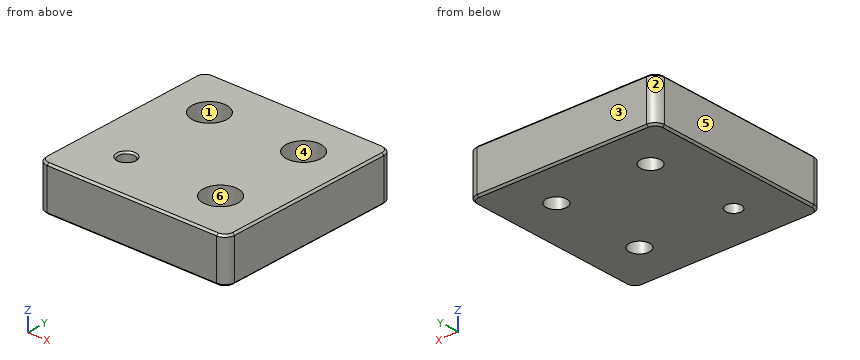
```python
from build123d import *

# Parameters (mm, degrees)
SKETCH1_W                                           = 60
SKETCH1_H                                           = 60
BOSS_EXTRUDE1_DEPTH                                 = 14
CBORE_FOR_M6_HEX_SOCKET_HEAD_CAP_SCREW1_D           = 6.5
CBORE_FOR_M6_HEX_SOCKET_HEAD_CAP_SCREW1_CBORE_D     = 11
CBORE_FOR_M6_HEX_SOCKET_HEAD_CAP_SCREW1_CBORE_DEPTH = 8
M6_TAPPED_HOLE1_D                                   = 5
M6_TAPPED_HOLE1_CSINK_D                             = 6.05
M6_TAPPED_HOLE1_CSINK_ANGLE                         = 90
FILLET1_R                                           = 3
CHAMFER1_SIZE                                       = 0.6


with BuildPart() as part:
    # Sketch1 → Boss-Extrude1 (new body)
    with BuildSketch(Plane.XY):
        Rectangle(SKETCH1_W, SKETCH1_H)
    extrude(amount=BOSS_EXTRUDE1_DEPTH)

    # CBORE for M6 Hex Socket Head Cap Screw1 (through all)
    with Locations(Plane.XY.offset(14)):
        with Locations((-15, 15), (15, 15), (15, -15)):
            CounterBoreHole(CBORE_FOR_M6_HEX_SOCKET_HEAD_CAP_SCREW1_D / 2, CBORE_FOR_M6_HEX_SOCKET_HEAD_CAP_SCREW1_CBORE_D / 2, CBORE_FOR_M6_HEX_SOCKET_HEAD_CAP_SCREW1_CBORE_DEPTH)

    # M6 Tapped Hole1 (through all)
    with Locations(Plane.XY.offset(14)):
        with Locations((-15, -15)):
            CounterSinkHole(M6_TAPPED_HOLE1_D / 2, M6_TAPPED_HOLE1_CSINK_D / 2, counter_sink_angle=M6_TAPPED_HOLE1_CSINK_ANGLE)

    # Fillet1
    fillet1_edges = [part.edges().sort_by_distance(p)[0] for p in [
        (-30, 30, 7),
        (30, 30, 7),
        (30, -30, 7),
        (-30, -30, 7),
    ]]
    fillet(fillet1_edges, radius=FILLET1_R)

    # Chamfer1
    chamfer1_edges = [part.edges().sort_by_distance(p)[0] for p in [
        (-30, 0, 0),
        (-30, 0, 14),
        (0, 30, 0),
        (30, 0, 0),
        (0, -30, 0),
        (-29.121320344, -29.121320344, 0),
        (29.121320344, -29.121320344, 0),
        (29.121320344, 29.121320344, 0),
        (-29.121320344, 29.121320344, 0),
        (0, 30, 14),
        (0, -30, 14),
        (30, 0, 14),
        (-29.121320344, -29.121320344, 14),
        (29.121320344, -29.121320344, 14),
        (29.121320344, 29.121320344, 14),
        (-29.121320344, 29.121320344, 14),
    ]]
    chamfer(chamfer1_edges, length=CHAMFER1_SIZE)


solid = part.part
```
Work out the finished part from the listing and answer in its coordinate system (mm). Face numbers are marked on the shaded views. A direction names the side the tool comes from. Round coordinates to 2 decimals unless told otherwise and drop trailing zeros. Loops run counter-clockwise (first coordinate to the right, second up) from the corner with the lowest first, then second, coordinate; pieces in that order, holes last.
(1) The mould has two halves that part along X. Classify the marked faces 3, 4, 5 and 6: pulls with the +X half, pulls with the -X half, needs draft (parallel to the pull), parting line crosses it, or undercut.
Computed values:
face 3: needs draft
face 4: undercut
face 5: pulls with the -X half
face 6: undercut
(2) Each of these flat-tipped pins is pushed along its axis until it touches: P1, Ø12, axis at x = 16, y = -13, coming from the +Z side; P2, Ø3.5, axis at x = -13, y = 15.5, coming from the +Z side. Where does it stop, or does it pass through?
Computed values:
P1: stops at z = 14
P2: stops at z = 6
(3) The part is cut by section A-A, the plane y = 15. Give the vertices of the cut face in (x, z), and give its area (3 significant figures).
Computed values:
outline: (-30, 0.6) - (-29.4, 0) - (-18.25, 0) - (-18.25, 6) - (-20.5, 6) - (-20.5, 14) - (-29.4, 14) - (-30, 13.4) - close; (-11.75, 0) - (11.75, 0) - (11.75, 6) - (9.5, 6) - (9.5, 14) - (-9.5, 14) - (-9.5, 6) - (-11.75, 6) - close; (18.25, 0) - (29.4, 0) - (30, 0.6) - (30, 13.4) - (29.4, 14) - (20.5, 14) - (20.5, 6) - (18.25, 6) - close
area: 585 mm2
(4) Find the intervals of material crossed by L1, parallel to Y at x = 15, z = 12; L2, parallel to Y at x = 15, z = 3.05; L3, parallel to X at y = 14, z = 6.5, in increasing order.
Computed values:
L1: y = -30 to -20.5, -9.5 to 9.5, 20.5 to 30
L2: y = -30 to -18.25, -11.75 to 11.75, 18.25 to 30
L3: x = -30 to -20.41, -9.59 to 9.59, 20.41 to 30
(5) For the marked faces 1 and 2, determine the directions among +Z, -Z, +X, -X, +Y, -Y from which every point of the face is accessible in a straight line to the end or side of a thin tool.
Computed values:
face 1: +Z
face 2: +Z, -Z, -X, +Y
(6) The part is cut by section C-C, the plane z = 12.5. Give the vertices of the cut face in (x, y), and give its area (3 significant figures).
Computed values:
outline: (-30, -27) arc R3 ccw to (-27, -30) - (27, -30) arc R3 ccw to (30, -27) - (30, 27) arc R3 ccw to (27, 30) - (-27, 30) arc R3 ccw to (-30, 27) - close; hole circle Ø11 at (-15, 15); hole circle Ø5 at (-15, -15); hole circle Ø11 at (15, -15); hole circle Ø11 at (15, 15)
area: 3,290 mm2
(7) The part is cut by section D-D, the plane x = -15. Give the vertices of the cut face in (y, z) (3 decimals).
Computed values:
outline: (-30, 0.6) - (-29.4, 0) - (-17.5, 0) - (-17.5, 13.475) - (-18.025, 14) - (-29.4, 14) - (-30, 13.4) - close; (-12.5, 0) - (11.75, 0) - (11.75, 6) - (9.5, 6) - (9.5, 14) - (-11.975, 14) - (-12.5, 13.475) - close; (18.25, 0) - (29.4, 0) - (30, 0.6) - (30, 13.4) - (29.4, 14) - (20.5, 14) - (20.5, 6) - (18.25, 6) - close
